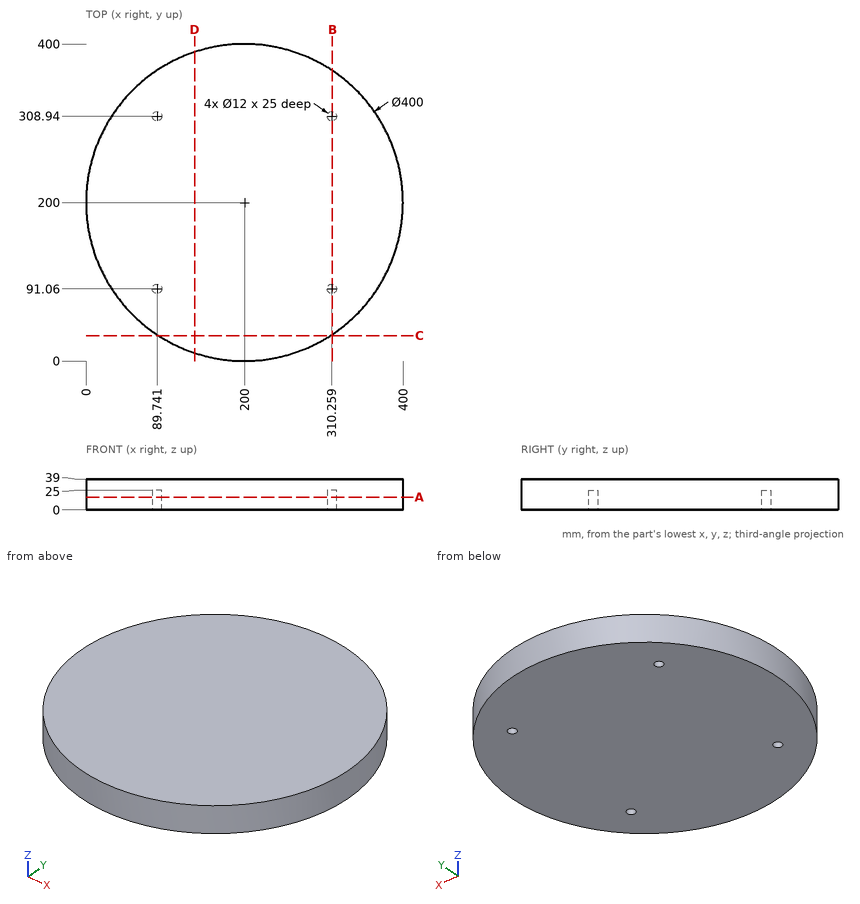
Can you work these out from the drawing? Everything is in mm from the part's minimum corner. Round coordinates to 2 decimals unless told otherwise and drop trailing zeros. Order: outer loops, then holes, each group sorted by start corner. A loop starts at its lowest first (then second) coordinate and runs counter-clockwise, first axis right, second up.
(1) If we section it at C-C (y = 32): Please give me the cut outline in (x, z), plus the area to 3 significant figures.
Results are:
outline: (91.48, 0) - (308.52, 0) - (308.52, 39) - (91.48, 39) - close
area: 8,460 mm2
(2) If I drill on L1, parallel to Y at x = 91, z = 13.5; L2, parallel to X at y = 212.5, z = 30; L3, parallel to Y at x = 252.5, z = 21, over which ranges is the centre line in solid material (lowest first)?
Results are:
L1: y = 32.31 to 85.19, 96.93 to 303.07, 314.81 to 367.69
L2: x = 0.39 to 399.61
L3: y = 7.01 to 392.99
(3) If we section it at B-B (x = 311): Please give me the cut outline in (y, z).
Results are:
outline: (33.63, 0) - (85.11, 0) - (85.11, 25) - (97.01, 25) - (97.01, 0) - (302.99, 0) - (302.99, 25) - (314.89, 25) - (314.89, 0) - (366.37, 0) - (366.37, 39) - (33.63, 39) - close
(4) I'm going to push flat-ended pins straight in: pin 1 (11 mm diameter, centred on x = 89.74, y = 308.94, fed in from -Z); pin 2 (1 mm diameter, centred on x = 249, z = 21, fed in from -Y); pin 3 (3 mm diameter, centred on x = 256, z = 18, fed in from +Y). Where does each tip first touch, or does it pass through?
Results are:
pin 1: stops at z = 25
pin 2: stops at y = 5.97
pin 3: stops at y = 392.43
(5) If we section it at D-D (x = 137): Please give me the cut outline in (y, z), plus the area to 3 significant figures.
Results are:
outline: (10.18, 0) - (389.82, 0) - (389.82, 39) - (10.18, 39) - close
area: 14,800 mm2
(6) If we section it at A-A (z = 16): Please give me the cut outline in (x, y).
Results are:
outline: circle Ø400 at (200, 200); hole circle Ø12 at (89.74, 91.06); hole circle Ø12 at (89.74, 308.94); hole circle Ø12 at (310.26, 91.06); hole circle Ø12 at (310.26, 308.94)
